Input: part model. Units: mm. Frame: model coordinates. Face numbers are marked on the shaded views. A direction names the side the tool comes from. Coordinates: 2 decimals unless noted, no trailing zeros. Loops run counter-clockwise (first coordinate to the right, second up) from the corner with the lowest first, then second, coordinate; pieces in that order, holes last.
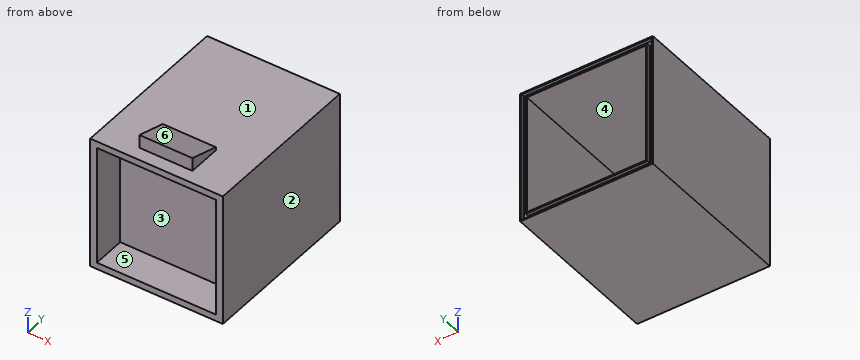
Autodesk Inventor part; units mm, degrees
ref_plane "YZ Plane" through (0, 0, 0) normal (1, 0, 0) x (0, 1, 0)
ref_plane "XZ Plane" through (0, 0, 0) normal (0, 1, 0) x (-1, 0, 0)
ref_plane "XY Plane" through (0, 0, 0) normal (0, 0, 1) x (1, 0, 0)
sketch "Skizze1" plane through (0, 0, 0) normal (0, 0, 1) x (1, 0, 0)
  line L0 (-140, 0) -> (140, 0)
  line L1 (0, -140) -> (0, 140)
  line L2 (-100, 100) -> (100, 100)
  line L3 (100, 100) -> (100, -100)
  line L4 (100, -100) -> (-100, -100)
  line L5 (-100, -100) -> (-100, 100)
  point P0 (0, 0)
  dimension "d0" = 200
  dimension "d1" = 200
  dimension "d2" = 100
  dimension "d3" = 100
extrude "Extrusion1" add sketch "Skizze1" along normal blind 200
sketch "Skizze2" plane through (-100, 100, 0) normal (0, 1, 0) x (1, 0, 0)
  line L0 (10, -10) -> (190, -10)
  line L1 (190, -10) -> (190, -190)
  line L2 (190, -190) -> (10, -190)
  line L3 (10, -190) -> (10, -10)
  line L4 (0, 0) -> (0, -200)
  line L5 (200, 0) -> (200, -200)
  line L6 (200, -200) -> (0, -200)
  line L7 (200, 0) -> (0, 0)
  point P0 (100, 0)
  dimension "d6" = 10
  dimension "d7" = 10
  dimension "d8" = 10
  dimension "d9" = 10
extrude "Extrusion2" cut sketch "Skizze2" against normal blind 190 contours L0 L1 L2 L3
sketch "Skizze3" plane through (-100, 100, 0) normal (0, 1, 0) x (1, 0, 0)
  line L0 (2, -2) -> (198, -2)
  line L1 (198, -2) -> (198, -198)
  line L2 (198, -198) -> (2, -198)
  line L3 (2, -198) -> (2, -2)
  line L4 (8, -8) -> (192, -8)
  line L5 (192, -8) -> (192, -192)
  line L6 (192, -192) -> (8, -192)
  line L7 (8, -192) -> (8, -8)
  line L8 (0, 0) -> (0, -200)
  line L9 (10, -190) -> (10, -10)
  line L10 (190, -190) -> (10, -190)
  line L11 (200, -200) -> (0, -200)
  line L12 (190, -10) -> (190, -190)
  line L13 (200, 0) -> (200, -200)
  line L14 (200, 0) -> (0, 0)
  line L15 (10, -10) -> (190, -10)
  point P0 (100, 0)
  dimension "d12" = 2
  dimension "d13" = 2
  dimension "d14" = 2
  dimension "d15" = 2
  dimension "d16" = 2
  dimension "d17" = 2
  dimension "d18" = 2
  dimension "d19" = 2
extrude "Extrusion3" cut sketch "Skizze3" against normal blind 5 contours L0 L1 L2 L3
fillet "Rundung1" radius 0.5 8 edges at (0, 100, 2) (0, 100, 8) (98, 100, 100) (92, 100, 100) (0, 100, 192) (0, 100, 198) (-98, 100, 100) (-92, 100, 100)
sketch "Skizze5" plane through (-100, -90, 0) normal (0, 1, 0) x (1, 0, 0)
  line L0 (95, -95) -> (105, -95)
  line L1 (105, -95) -> (105, -105)
  line L2 (105, -105) -> (95, -105)
  line L3 (95, -105) -> (95, -95)
  line L4 (200, 0) -> (0, 0)
  line L5 (0, 0) -> (0, -200)
  point P0 (100, 0)
  dimension "d24" = 10
  dimension "d25" = 10
  dimension "d26" = 95
  dimension "d27" = 95
extrude "Extrusion4" cut sketch "Skizze5" against normal blind 7
sketch "Skizze6" plane through (-100, -100, 0) normal (0, -1, 0) x (1, 0, 0)
  line L0 (10, 190) -> (190, 190)
  line L1 (190, 190) -> (190, 10)
  line L2 (190, 10) -> (10, 10)
  line L3 (10, 10) -> (10, 190)
  line L4 (0, 200) -> (200, 200)
  line L5 (200, 0) -> (200, 200)
  line L6 (0, 0) -> (200, 0)
  line L7 (0, 0) -> (0, 200)
  point P0 (100, 0)
  dimension "d30" = 10
  dimension "d31" = 10
  dimension "d32" = 10
  dimension "d33" = 10
extrude "Extrusion5" add sketch "Skizze6" along normal blind 50
sketch "Skizze7" plane through (0, 0, 200) normal (0, 0, 1) x (1, 0, 0)
  line L0 (-40, -130) -> (40, -130)
  line L1 (40, -130) -> (40, -80)
  line L2 (40, -80) -> (-40, -80)
  line L3 (-40, -80) -> (-40, -130)
  line L4 (100, -150) -> (-100, -150)
  line L5 (-100, 100) -> (-100, -150)
  point P0 (0, 0)
  dimension "d36" = 50
  dimension "d37" = 80
  dimension "d38" = 20
  dimension "d39" = 60
extrude "Extrusion6" add sketch "Skizze7" along normal blind 20
sketch "Skizze9" plane through (-40, -130, 200) normal (-1, 0, 0) x (0, 0, 1)
  line L0 (20, 0) -> (20, 50)
  line L1 (20, 0) -> (5, 50)
  line L2 (0, 50) -> (20, 50)
  line L3 (0, 230) -> (0, -20)
  point P0 (-200, 130)
  dimension "d45" = 5
extrude "Extrusion7" cut sketch "Skizze9" against normal blind 200
fillet "Rundung2" radius 2 4 edges at (0, -90, 10) (90, -90, 100) (0, -90, 190) (-90, -90, 100)
chamfer "Fase1" distance 1 angle 45 4 edges at (0, -90, 95) (5, -90, 100) (0, -90, 105) (-5, -90, 100)
properties material "Acetalharz, Schwarz"
Item 1: Line query: L1, parallel to Z at x = -25.5, y = 9; L2, parallel to X at y = -136.5, z = 98.5; L3, parallel to Z at x = -15.5, y = -129. Output: solid intervals per line, ascending.
Result:
L1: z = 0 to 10, 190 to 200
L2: x = -100 to -90, 90 to 100
L3: z = 0 to 10, 190 to 219.7
Item 2: Reachability of the marked faces 4, 5 and 6 from +Z, -Z, +X, -X, +Y, -Y: full face, straight path, thin tool, end or side. Return the list, or none.
Result:
face 4: +Y
face 5: -Y
face 6: +Z, +X, -X, +Y
Item 3: Section query C-C (z = 22.5). Output: boundary loops of the cut face in (x, y), then the cut area to 3 significant figures.
Result:
outline: (-100, -150) - (-90, -150) - (-90, -100) - (90, -100) - (90, -150) - (100, -150) - (100, 100) - (98.5, 100) arc R0.5 ccw to (98, 99.5) - (98, 95) - (92, 95) - (92, 99.5) arc R0.5 ccw to (91.5, 100) - (90, 100) - (90, -88) arc R2 cw to (88, -90) - (-88, -90) arc R2 cw to (-90, -88) - (-90, 100) - (-91.5, 100) arc R0.5 ccw to (-92, 99.5) - (-92, 95) - (-98, 95) - (-98, 99.5) arc R0.5 ccw to (-98.5, 100) - (-100, 100) - close
area: 6,740 mm2
Item 4: Section query B-B (x = -58). Output: boundary loops of the cut face in (y, z), then the cut area to 3 significant figures.
Result:
outline: (-150, 0) - (100, 0) - (100, 1.5) arc R0.5 ccw to (99.5, 2) - (95, 2) - (95, 8) - (99.5, 8) arc R0.5 ccw to (100, 8.5) - (100, 10) - (-88, 10) arc R2 cw to (-90, 12) - (-90, 188) arc R2 cw to (-88, 190) - (100, 190) - (100, 191.5) arc R0.5 ccw to (99.5, 192) - (95, 192) - (95, 198) - (99.5, 198) arc R0.5 ccw to (100, 198.5) - (100, 200) - (-150, 200) - (-150, 190) - (-100, 190) - (-100, 10) - (-150, 10) - close
area: 6,740 mm2
Item 5: Mould query, pull axis X, two halves, no side actions, for the marked faces 1, 2 and 3. Classes: +X half, -X half, draft (parallel to the pull), parting line (faces both ways), or undercut.
Result:
face 1: draft
face 2: +X half
face 3: undercut
Item 6: Contact query for flat-ended pins moving along their axis: P1, Ø2, axis at x = -19.5, z = 139, coming from the +Y side; P2, Ø16, axis at y = -103, z = 214.5, coming from the -X side; P3, Ø1.5, axis at x = 68.5, z = 124, coming from the -Y side. Output: stop coordinate, or through.
Result:
P1: stops at y = -90
P2: stops at x = -40
P3: stops at y = -100
Item 7: Section query A-A (y = -1). Output: boundary loops of the cut face in (x, z), then the cut area to 3 significant figures.
Result:
outline: (-100, 0) - (100, 0) - (100, 200) - (-100, 200) - close; hole (-90, 10) - (90, 10) - (90, 190) - (-90, 190) - close
area: 7,600 mm2
